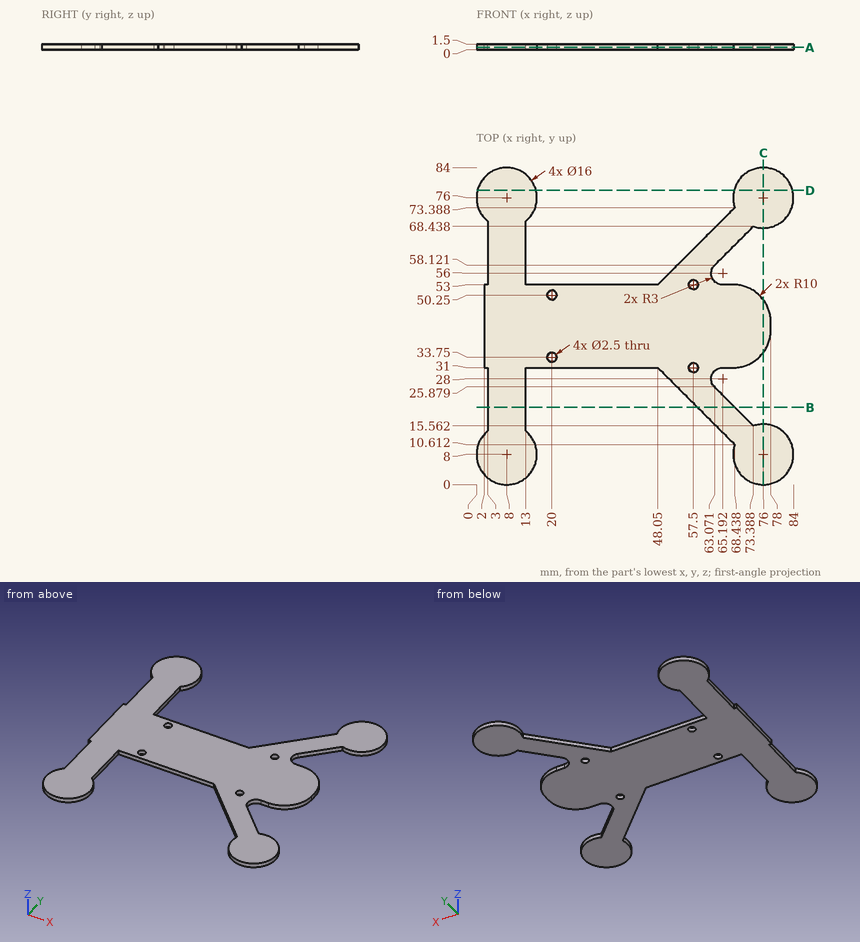
Input: dimensioned drawing with shaded views. Units: mm. Origin: part minimum x, y, z. Coordinates: 2 decimals unless noted, no trailing zeros. Loops run counter-clockwise (first coordinate to the right, second up) from the corner with the lowest first, then second, coordinate; pieces in that order, holes last. Notation, with made-up numbers: (23, 49.5) -> (68, 49.5) arc R38 ccw to (68, 87.5) -> close; hole circle Ø9 at (38.25, 6). An arc over 180 degrees is marked (long way). Use a Markdown table: item, result. Add a question column.
(1) Pin query (flat end, axial travel): pin 1 Ø4 at (x, y) = (66.5, 57.5) entering from +Z; pin 2 Ø0.5 at (x, z) = (2.5, 1) entering from -Y (1 decimal); pin 3 Ø0.8 at (y, z) = (26, 0.5) entering from +X; pin 4 Ø0.8 at (x, z) = (66, 0.5) entering from -Y. Return the tip coordinate at first contact, or that it passes through.
(2) Section query A-A, the plane z = 0.6. State how many separate pieces and enclosed holes the cut face has, plus the area to 3 significant figures.
(3) Section query D-D, the plane y = 78. Return loops of the section in (x, z).
(4) Section query C-C, the plane x = 76. Return loops of the section in (y, z).
(5) Section query B-B, the plane y = 20.5. Return loops of the section in (x, z).
(6) Line query: line 1 along Y through (x, z) = (20, 1.1); line 2 along Y through (x, z) = (57.5, 0.3); line 3 along X through (y, z) = (7.5, 1.4) (1 decimal). Output: solid intervals per line, ascending.
Answer:
| question | item | result |
|---|---|---|
| 1 | pin 1 | passes through |
| 1 | pin 2 | stops at y = 2 |
| 1 | pin 3 | stops at x = 63.35 |
| 1 | pin 4 | stops at y = 12.65 |
| 2 | separate pieces | 1 |
| 2 | enclosed holes | 4 |
| 2 | area | 3,090 mm^2 |
| 3 | outline | (0.25, 0) -> (15.75, 0) -> (15.75, 1.5) -> (0.25, 1.5) -> close; (68.25, 0) -> (83.75, 0) -> (83.75, 1.5) -> (68.25, 1.5) -> close |
| 4 | outline | (0, 0) -> (16, 0) -> (16, 1.5) -> (0, 1.5) -> close; (35, 0) -> (49, 0) -> (49, 1.5) -> (35, 1.5) -> close; (68, 0) -> (84, 0) -> (84, 1.5) -> (68, 1.5) -> close |
| 5 | outline | (3, 0) -> (13, 0) -> (13, 1.5) -> (3, 1.5) -> close; (58.55, 0) -> (68.45, 0) -> (68.45, 1.5) -> (58.55, 1.5) -> close |
| 6 | line 1 | y = 31 to 32.5, 35 to 49, 51.5 to 53 |
| 6 | line 2 | y = 21.55 to 29.75, 32.25 to 51.75, 54.25 to 62.45 |
| 6 | line 3 | x = 0 to 16, 68 to 84 |
